For this review, use the dimensioned drawing (mm, ordinates from the lowest corner) and the shaded views. A direction names the side the tool comes from. Give positions to 0.01 mm unless a question says otherwise; leave off trailing zeros. Order: outer loops, then holes, each group sorted by start corner. A loop starts at its lowest first (then second) coordinate and runs counter-clockwise, first axis right, second up. Notation, with made-up numbers: M -37,82 L 10,82 A22 ccw 10,92 Z; hole C 62.25,-26 d3. An arc over 180 degrees is marked long. One line per question, with ' | ' between items. Start each with the question number.
1. Wall thickness on L1, parallel to Z at x = 32.5, y = 46; L2, parallel to X at y = 36, z = 9; L3, parallel to Z at x = 6.5, y = 31: over which ranges is each line inside the solid? List them lowest first.
2. We need section D-D on x = 36. Write out the cut boundary in (y, z).
3. We need section C-C on z = 8.5. Write out the cut boundary in (x, y), then the cut area to 3 significant figures.
4. We need section B-B on x = 47. Write out the cut boundary in (y, z), then the cut area to 3 significant figures.
5. Insertion check: P1, Ø12, axis at x = 36, z = 12.5, coming from the -Y side; P2, Ø1.6, axis at y = 13.5, z = 1.5, coming from the +X side; P3, Ø7, axis at x = 14.5, z = 31, coming from the -Y side; P4, Ø1, axis at x = 34.5, y = 19, coming from the +Z side. Each pin has a flat end and moves straight along its axis. Give the tip position at first contact, or say it passes through.
6. We need section A-A on y = 9. Write out the cut boundary in (x, z), then the cut area to 3 significant figures.
7. For the marked faces 1 and 2, list the 3-axis set-ups (+Z, -Z, +X, -X, +Y, -Y) from which the entire face can be reached by the end or side of a thin tool; tool diameter is ignored.
8. The part is to be moulded in two halves that separate along X. For the marked faces 3, 4, 5 and 6, say which applies: +X half, -X half, draft (parallel to the pull), parting line (faces both ways), or undercut.
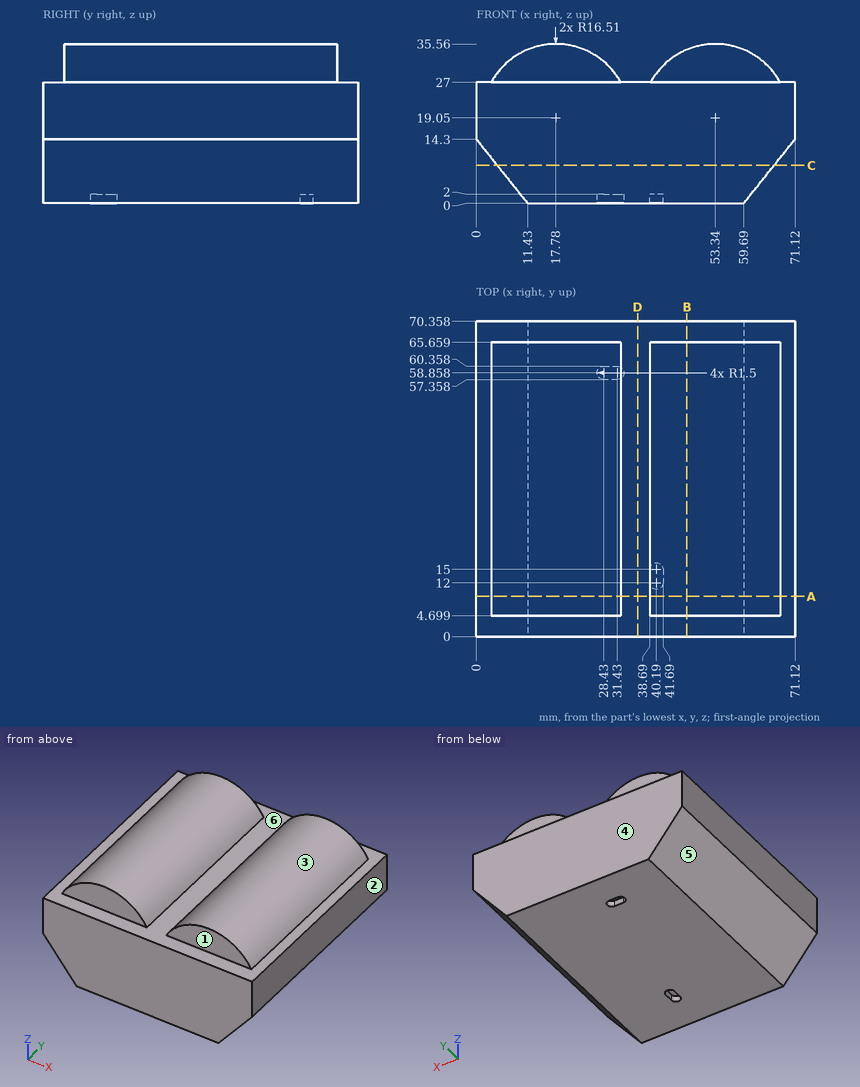
Entries:
1) L1: z = 0 to 27 | L2: x = 4.24 to 66.88 | L3: z = 6.17 to 31.11
2) outline: M 0,0 L 70.36,0 L 70.36,27 L 0,27 Z
3) outline: M 4.64,0 L 66.48,0 L 66.48,70.36 L 4.64,70.36 Z | area: 4,350 mm^2
4) outline: M 0,0 L 70.36,0 L 70.36,27 L 65.66,27 L 65.66,34.29 L 4.7,34.29 L 4.7,27 L 0,27 Z | area: 2,340 mm^2
5) P1: stops at y = 0 | P2: stops at x = 61.53 | P3: stops at y = 4.7 | P4: stops at z = 27
6) outline: M 0,14.3 L 11.43,0 L 59.69,0 L 71.12,14.3 L 71.12,27 L 67.81,27 A16.51 ccw 38.87,27 L 32.25,27 A16.51 ccw 3.31,27 L 0,27 Z | area: 2,110 mm^2
7) face 1: +Z, +X, -X, -Y | face 2: +Z, -Z, +X, +Y, -Y
8) face 3: undercut | face 4: draft | face 5: -X half | face 6: undercut
